Geometry check sheet. Reference: the model listing, model coordinates, mm. Face numbers are marked on the shaded views. A direction names the side the tool comes from. Coordinates: 2 decimals unless noted, no trailing zeros. Loops run counter-clockwise (first coordinate to the right, second up) from the corner with the lowest first, then second, coordinate; pieces in that order, holes last. Notation, with made-up numbers: (-1, 67) - (33, 67) arc R26 ccw to (33, 87) - close; hole circle Ø9 at (9, 74.5). An arc over 180 degrees is marked (long way). One line per item, written item: value.
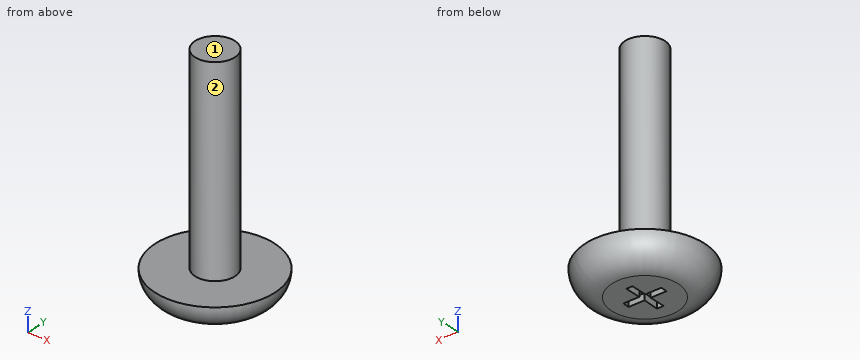
from build123d import *

# Parameters (mm, degrees)
SKETCH1_R           = 4.5
BOSS_EXTRUDE1_DEPTH = 2
FILLET1_R           = 2
CUT_EXTRUDE1_DEPTH  = 0.5
SKETCH3_R           = 1.5
BOSS_EXTRUDE2_DEPTH = 15


with BuildPart() as part:
    # Sketch1 → Boss-Extrude1 (new body)
    with BuildSketch(Plane.XY):
        Circle(SKETCH1_R)
    extrude(amount=BOSS_EXTRUDE1_DEPTH)

    # Fillet1
    fillet1_edges = [part.edges().sort_by_distance(p)[0] for p in [
        (-4.5, 0, 0),
    ]]
    fillet(fillet1_edges, radius=FILLET1_R - 0.0001)  # a hair under: the kernel refuses the full size

    # Sketch2 → Cut-Extrude1 (cut)
    with BuildSketch(Plane(origin=(0, 0, 0), x_dir=(-1, 0, 0), z_dir=(0, 0, -1))):
        Polygon((0.230798636, -0.25), (0.230798636, -1.45), (-0.269201364, -1.45), (-0.230798636, -0.25), (-1.430798636, -0.25), (-1.430798636, 0.25), (-0.230798636, 0.25), (-0.230798636, 1.45), (0.230798636, 1.45), (0.230798636, 0.25), (1.430798636, 0.25), (1.430798636, -0.25), align=None)
    extrude(amount=-CUT_EXTRUDE1_DEPTH, mode=Mode.SUBTRACT)

    # Sketch3 → Boss-Extrude2 (add)
    with BuildSketch(Plane.XY.offset(2)):
        Circle(SKETCH3_R)
    extrude(amount=BOSS_EXTRUDE2_DEPTH)


solid = part.part
(1) Go/stop test with flat-tipped pins: pin 1 Ø1 at (x, z) = (1.5, 7) entering from +Y; pin 2 Ø0.6 at (y, z) = (-1, 0) entering from +X; pin 3 Ø2 at (x, y) = (-1.5, -3) entering from -Z; pin 4 Ø3 at (x, y) = (-3.5, -3.5) entering from +Z. Record where each tip stops, or that it passes through.
Reply:
pin 1: y = 1.12
pin 2: x = 3.42
pin 3: z = 0
pin 4: z = 2
(2) Access from +Z, -Z, +X, -X, +Y, -Y to the whole of each face (thin tool, end or side, straight path). Record for the marked faces 1 and 2.
Reply:
face 1: +Z, +X, -X, +Y, -Y
face 2: +Z
(3) Cross-section at C-C on z = 3.25. Record the cut outline in (x, y), and give its area (3 significant figures).
Reply:
outline: circle Ø3 at (0, 0)
area: 7.07 mm2
(4) Material ranges on probe 1 along Z at (x, y) = (-0.5, 2.25); probe 2 along Z at (x, y) = (1.25, 3); probe 3 along Y at (x, z) = (-3.25, 1), recorded low to high. Write a range as from..to.
Reply:
probe 1: 0..2
probe 2: 0.15..2
probe 3: -2.71..2.71
